Here's the drawing with two shaded views (mm, measured from the low corner). I have some questions. Coordinates: 2 decimals unless noted, no trailing zeros. Loops run counter-clockwise (first coordinate to the right, second up) from the corner with the lowest first, then second, coordinate; pieces in that order, holes last. Notation, with made-up numbers: (43, 67.25) -> (97, 67.25) arc R3 ccw to (97, 72.25) -> close; hole circle Ø4 at (-18.5, 27.25). An arc over 180 degrees is marked (long way). Answer as a JSON object with one key per item and string values. Group by question number.
Q1. I want a section at A-A on x = 29. Write out the boundary of the cut face in (y, z).
Q2. I want a section at D-D on y = 1.1. Write out the boundary of the cut face in (x, z), then the cut area to 3 significant figures.
Q3. Thinking about a two-plate mould opening in Y: for the marked faces 1 and 2, which applies, released by +Y, released by -Y, zero draft, split by the parting line, or undercut?
Q4. I want a section at B-B on x = 46. Write out the boundary of the cut face in (y, z), then the cut area to 4 significant figures.
Q5. I want a section at C-C on z = 25. Write out the boundary of the cut face in (x, y), then the cut area to 3 significant figures.
Q6. I need wall thicknesses on line 1 (X direction, y = 2.4, z = 25); line 2 (Z direction, x = 40, y = 0.55); line 3 (Z direction, x = 29.5, y = 1.4). Which ranges of each line are inside material? Lowest first, please.
Q7. I'm going to push flat-ended pins straight in: pin 1 (2.5 mm diameter, centred on x = 29, z = 25, fed in from -Y) (1 decimal); pin 2 (2 mm diameter, centred on x = 15, y = 1, fed in from -Z); pin 3 (2 mm diameter, centred on y = 2.5, z = 62.5, fed in from -X); pin 4 (2 mm diameter, centred on y = 2.5, z = 55, fed in from -X). Where does each tip first touch, or does it pass through?
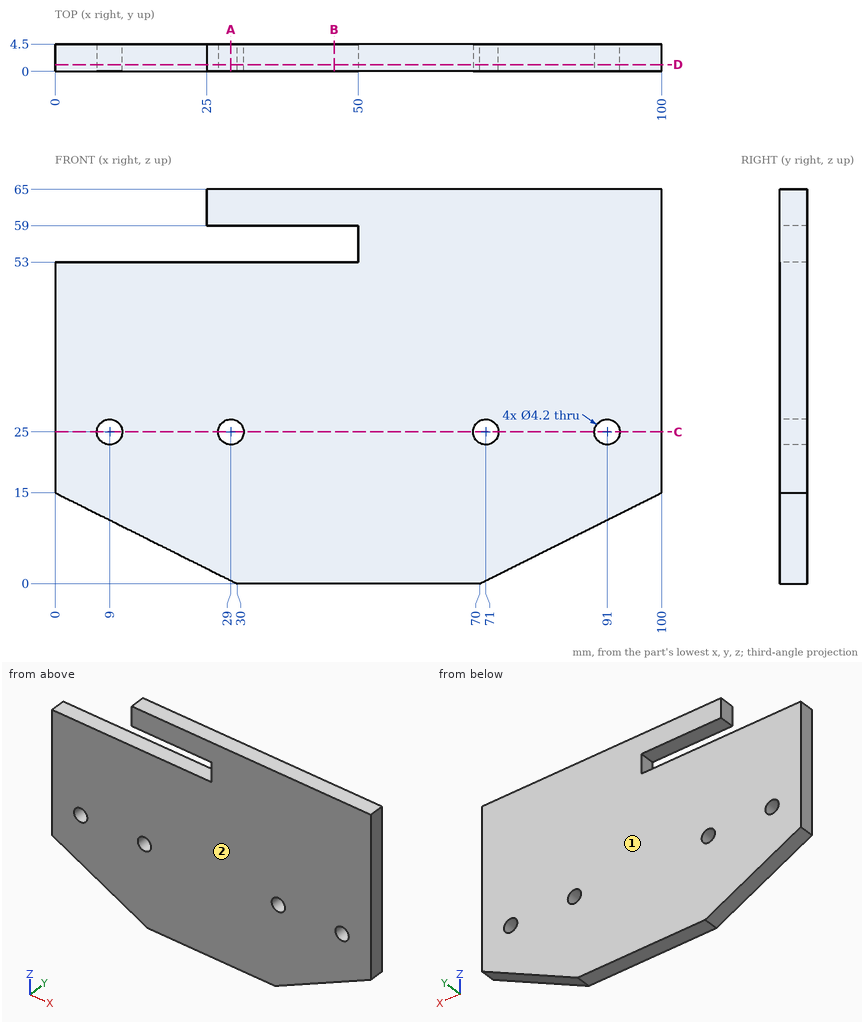
Result set:
{
 "1": {"outline": "(0, 0.5) -> (4.5, 0.5) -> (4.5, 22.9) -> (0, 22.9) -> close; (0, 27.1) -> (4.5, 27.1) -> (4.5, 53) -> (0, 53) -> close; (0, 59) -> (4.5, 59) -> (4.5, 65) -> (0, 65) -> close"},
 "2": {"outline": "(0, 15) -> (30, 0) -> (70, 0) -> (100, 15) -> (100, 65) -> (25, 65) -> (25, 59) -> (50, 59) -> (50, 53) -> (0, 53) -> close; hole circle Ø4.2 at (9, 25); hole circle Ø4.2 at (29, 25); hole circle Ø4.2 at (71, 25); hole circle Ø4.2 at (91, 25)", "area": "5,540 mm²"},
 "3": {"face 1": "released by +Y", "face 2": "released by -Y"},
 "4": {"outline": "(0, 0) -> (4.5, 0) -> (4.5, 53) -> (0, 53) -> close; (0, 59) -> (4.5, 59) -> (4.5, 65) -> (0, 65) -> close", "area": "265.5 mm²"},
 "5": {"outline": "(0, 0) -> (6.9, 0) -> (6.9, 4.5) -> (0, 4.5) -> close; (11.1, 0) -> (26.9, 0) -> (26.9, 4.5) -> (11.1, 4.5) -> close; (31.1, 0) -> (68.9, 0) -> (68.9, 4.5) -> (31.1, 4.5) -> close; (73.1, 0) -> (88.9, 0) -> (88.9, 4.5) -> (73.1, 4.5) -> close; (93.1, 0) -> (100, 0) -> (100, 4.5) -> (93.1, 4.5) -> close", "area": "374 mm²"},
 "6": {"line 1": "x = 0 to 6.9, 11.1 to 26.9, 31.1 to 68.9, 73.1 to 88.9, 93.1 to 100", "line 2": "z = 0 to 53, 59 to 65", "line 3": "z = 0.25 to 22.96, 27.04 to 53, 59 to 65"},
 "7": {"pin 1": "passes through", "pin 2": "stops at z = 7", "pin 3": "stops at x = 25", "pin 4": "stops at x = 50"}
}
